from build123d import *
from build123d.topology import SkipClean

# Parameters (mm, degrees)
SKETCH1_R            = 8.255
BOSS_EXTRUDE1_DEPTH  = 266.7
BOSS_EXTRUDE2_START  = 12.7
BOSS_EXTRUDE2_DEPTH  = 12.7
SKETCH5_R            = 3.175
CUT_EXTRUDE1_DEPTH   = 268.246525418
FILLET2_R            = 5.08
FILLET2_OF_MIRROR1_R = 5.08


with BuildPart() as part:
    # Sketch1 → Boss-Extrude1 (new body)
    with BuildSketch(Plane.YZ):
        with Locations(Location((0, 0, 0), (0, 0, 270))):
            Circle(SKETCH1_R)
    boss_extrude1 = extrude(amount=-BOSS_EXTRUDE1_DEPTH)

    # Sketch4 → Boss-Extrude2 (add)
    with SkipClean():  # the faces are left unmerged after this step: merging them gives an invalid solid
        with BuildSketch(Plane.YZ.offset(BOSS_EXTRUDE2_START)):
            with BuildLine():
                Line((-7.113903851, -4.187767543), (7.113903851, -4.187767543))
                ThreePointArc((7.113903851, -4.187767543), (6.098527778, -5.563540594), (4.821496361, -6.700611751))
                Line((4.821496361, -6.700611751), (-4.821496361, -6.700611751))
                ThreePointArc((-4.821496361, -6.700611751), (-6.098527778, -5.563540594), (-7.113903851, -4.187767543))
            make_face()
            with BuildLine():
                Line((-7.113903851, 4.187767543), (7.113903851, 4.187767543))
                ThreePointArc((7.113903851, 4.187767543), (6.098527778, 5.563540594), (4.821496361, 6.700611751))
                Line((4.821496361, 6.700611751), (-4.821496361, 6.700611751))
                ThreePointArc((-4.821496361, 6.700611751), (-6.098527778, 5.563540594), (-7.113903851, 4.187767543))
            make_face()
        boss_extrude2 = extrude(amount=-BOSS_EXTRUDE2_DEPTH)

    # Sketch5 → Cut-Extrude1 (cut, through all)
    with SkipClean():  # the faces are left unmerged after this step: merging them gives an invalid solid
        with BuildSketch(Plane.XY.offset(6.700611751)):
            with Locations((6.35, 0)):
                Circle(SKETCH5_R)
        cut_extrude1 = extrude(amount=-CUT_EXTRUDE1_DEPTH, mode=Mode.SUBTRACT)

    # Fillet2
    # the kernel refuses this fillet: 5.08 mm, written as the material it takes off along each edge
    with BuildSketch(Plane(origin=(12.7, 0, 0), x_dir=(0, 0.7924229506159141, -0.6099720217658908), z_dir=(0, 0.6099720217658908, 0.7924229506159141))) as fillet2_piece_1:
        with BuildLine():
            CenterArc((8.255 - FILLET2_R, FILLET2_R), FILLET2_R, 270, 90)
            Line((8.255 - FILLET2_R, 0), (8.255, 0))
            Line((8.255, 0), (8.255, FILLET2_R))
        make_face()
    revolve(axis=Axis((12.7, 0, 0), (-1, 0, 0)), revolution_arc=200.07814468, mode=Mode.SUBTRACT)
    with BuildSketch(Plane(origin=(12.7, 0, 0), x_dir=(0, 0.534859378845264, 0.8449410895803674), z_dir=(0, -0.8449410895803674, 0.534859378845264))) as fillet2_piece_2:
        with BuildLine():
            CenterArc((8.255 - FILLET2_R, FILLET2_R), FILLET2_R, 270, 90)
            Line((8.255 - FILLET2_R, 0), (8.255, 0))
            Line((8.255, 0), (8.255, FILLET2_R))
        make_face()
    revolve(axis=Axis((12.7, 0, 0), (-1, 0, 0)), revolution_arc=200.07814468, mode=Mode.SUBTRACT)
    with BuildSketch(Plane(origin=(12.7, 0, 0), x_dir=(0, 0.7924229506159125, 0.6099720217658933), z_dir=(0, 0.6099720217658933, -0.7924229506159125))) as fillet2_piece_3:
        with BuildLine():
            CenterArc((8.255 - FILLET2_R, -FILLET2_R), FILLET2_R, 0, 90)
            Line((8.255 - FILLET2_R, 0), (8.255, 0))
            Line((8.255, 0), (8.255, -FILLET2_R))
        make_face()
    revolve(axis=Axis((12.7, 0, 0), (1, 0, 0)), revolution_arc=200.07814468, mode=Mode.SUBTRACT)
    with BuildSketch(Plane(origin=(12.7, 0, 0), x_dir=(0, 0.534859378845264, -0.8449410895803674), z_dir=(0, -0.8449410895803674, -0.534859378845264))) as fillet2_piece_4:
        with BuildLine():
            CenterArc((8.255 - FILLET2_R, -FILLET2_R), FILLET2_R, 0, 90)
            Line((8.255 - FILLET2_R, 0), (8.255, 0))
            Line((8.255, 0), (8.255, -FILLET2_R))
        make_face()
    revolve(axis=Axis((12.7, 0, 0), (1, 0, 0)), revolution_arc=200.07814468, mode=Mode.SUBTRACT)

    # Mirror1: Boss-Extrude1, Boss-Extrude2, Cut-Extrude1 across plane
    add(boss_extrude1.mirror(Plane(origin=(-133.35, 0, 0), x_dir=(0, 0, 1), z_dir=(1, 0, 0))))
    add(boss_extrude2.mirror(Plane(origin=(-133.35, 0, 0), x_dir=(0, 0, 1), z_dir=(1, 0, 0))))
    add(cut_extrude1.mirror(Plane(origin=(-133.35, 0, 0), x_dir=(0, 0, 1), z_dir=(1, 0, 0))), mode=Mode.SUBTRACT)

    # Fillet2 of Mirror1
    # the kernel refuses this fillet: 5.08 mm, written as the material it takes off along each edge
    with BuildSketch(Plane(origin=(-279.4, 0, 0), x_dir=(0, 0.7924229506159141, -0.6099720217658908), z_dir=(0, 0.6099720217658908, 0.7924229506159141))) as fillet2_of_mirror1_piece_1:
        with BuildLine():
            CenterArc((8.255 - FILLET2_OF_MIRROR1_R, -FILLET2_OF_MIRROR1_R), FILLET2_OF_MIRROR1_R, 0, 90)
            Line((8.255 - FILLET2_OF_MIRROR1_R, 0), (8.255, 0))
            Line((8.255, 0), (8.255, -FILLET2_OF_MIRROR1_R))
        make_face()
    revolve(axis=Axis((-279.4, 0, 0), (-1, 0, 0)), revolution_arc=200.07814468, mode=Mode.SUBTRACT)
    with BuildSketch(Plane(origin=(-279.4, 0, 0), x_dir=(0, 0.534859378845264, 0.8449410895803674), z_dir=(0, -0.8449410895803674, 0.534859378845264))) as fillet2_of_mirror1_piece_2:
        with BuildLine():
            CenterArc((8.255 - FILLET2_OF_MIRROR1_R, -FILLET2_OF_MIRROR1_R), FILLET2_OF_MIRROR1_R, 0, 90)
            Line((8.255 - FILLET2_OF_MIRROR1_R, 0), (8.255, 0))
            Line((8.255, 0), (8.255, -FILLET2_OF_MIRROR1_R))
        make_face()
    revolve(axis=Axis((-279.4, 0, 0), (-1, 0, 0)), revolution_arc=200.07814468, mode=Mode.SUBTRACT)
    with BuildSketch(Plane(origin=(-279.4, 0, 0), x_dir=(0, 0.7924229506159125, 0.6099720217658933), z_dir=(0, 0.6099720217658933, -0.7924229506159125))) as fillet2_of_mirror1_piece_3:
        with BuildLine():
            CenterArc((8.255 - FILLET2_OF_MIRROR1_R, FILLET2_OF_MIRROR1_R), FILLET2_OF_MIRROR1_R, 270, 90)
            Line((8.255 - FILLET2_OF_MIRROR1_R, 0), (8.255, 0))
            Line((8.255, 0), (8.255, FILLET2_OF_MIRROR1_R))
        make_face()
    revolve(axis=Axis((-279.4, 0, 0), (1, 0, 0)), revolution_arc=200.07814468, mode=Mode.SUBTRACT)
    with BuildSketch(Plane(origin=(-279.4, 0, 0), x_dir=(0, 0.534859378845264, -0.8449410895803674), z_dir=(0, -0.8449410895803674, -0.534859378845264))) as fillet2_of_mirror1_piece_4:
        with BuildLine():
            CenterArc((8.255 - FILLET2_OF_MIRROR1_R, FILLET2_OF_MIRROR1_R), FILLET2_OF_MIRROR1_R, 270, 90)
            Line((8.255 - FILLET2_OF_MIRROR1_R, 0), (8.255, 0))
            Line((8.255, 0), (8.255, FILLET2_OF_MIRROR1_R))
        make_face()
    revolve(axis=Axis((-279.4, 0, 0), (1, 0, 0)), revolution_arc=200.07814468, mode=Mode.SUBTRACT)


solid = part.part
Source: CAD feature listing. Evaluate the final solid. Frame: model axes, mm. A direction names the side the tool comes from. Coordinates: 2 decimals unless noted, no trailing zeros. Order: outer loops, then holes, each group sorted by start corner. A loop starts at its lowest first (then second) coordinate and runs counter-clockwise, first axis right, second up. Notation, with made-up numbers: M 55.25,69.5 L 95.25,69.5 A13 ccw 95.25,78.5 Z; hole C 39,10 d8. An arc over 180 degrees is marked long. Write each question's results on one line, items separated by ' | '. Start each with the question number.
Item 1: Set-up query: faces 1 (the face through (5, -3.3, 4.188)), 2 (the face through (3, -1, -6.701)), 3 (the face through (-270, -2, -4.188)). Return all of +Z, -Z, +X, -X, +Y, -Y with unobstructed straight access to the full face (end or side cutting, diameter ignored); none if empty.
Item 2: Cut plane B-B (z = 0). Return loops of the section in (x, y) (3 decimals), and give its area (3 significant figures).
Item 3: Line query: probe 1 along X at (y, z) = (-2.5, 3.75); probe 2 along Y at (x, z) = (-273.05, 6.25) (3 decimals); probe 3 along Y at (x, z) = (-206.5, -4.75). Output: solid intervals per line, ascending.
Item 4: Draft query along Y for faces 4 (the face through (-269.9, 1.1, 6.701)), 5 (the face through (-270.53, -1.93, 5.46)). Return one class per face: pulls with the +Y half, pulls with the -Y half, needs draft (parallel to the pull), parting line crosses it, or undercut.
Item 5: First-contact query: pin 1 Ø0.8 at (y, z) = (0.5, 7.5) entering from -X; pin 2 Ø7.5 at (x, y) = (-273.05, 0) entering from +Z; pin 3 Ø2 at (x, y) = (-248.5, -5.5) entering from -Z. Flat tips, straight axial feed; report the tip coordinate or a pass-through.
Item 6: Cut plane C-C (x = -197.5). Return loops of the section in (y, z) (3 decimals).
Item 7: Cut plane A-A (y = 0). Count the separate pieces of the cut face and the enclosed holes in it, and give its area (3 significant figures).
Checked values:
1) face 1: +X, +Y, -Y | face 2: -Z, +X, +Y, -Y | face 3: -X, +Y, -Y
2) outline: M -266.7,-8.255 L 0,-8.255 L 0,8.255 L -266.7,8.255 Z | area: 4,400 mm2
3) probe 1: x = -266.7 to 0 | probe 2: y = -5.393 to -3.175, 3.175 to 5.393 | probe 3: y = -6.75 to 6.75
4) face 4: needs draft | face 5: undercut
5) pin 1: stops at x = -266.7 | pin 2: stops at z = 6.7 | pin 3: stops at z = -6.92
6) outline: C 0,0 d16.51
7) separate pieces: 5 | enclosed holes: 0 | area: 4,460 mm2
